```python
from build123d import *

# Parameters (mm, degrees)
SKETCH2_R           = 3
BOSS_EXTRUDE1_DEPTH = 16
CHAMFER1_SIZE       = 1.9304
CHAMFER1_SIZE2      = 10.947842425
FILLET2_R           = 0.7112
SKETCH3_R           = 3.25
BOSS_EXTRUDE2_DEPTH = 2.5
SKETCH4_W           = 71.5000084
SKETCH4_H           = 6.5
BOSS_EXTRUDE3_DEPTH = 0.75
LPATTERN1_START     = 15.124999972
LPATTERN1_OUTLINE_R = 3.25
LPATTERN1_DEPTH     = 0.875000028
SKETCH5_W           = 83
SKETCH5_H           = 9
BOSS_EXTRUDE4_DEPTH = 0.7


# Read off the part's stored shape, not the designer's step: LPattern1
with BuildPart() as part:
    # Sketch2 → Boss-Extrude1 (new body)
    with BuildSketch(Plane(origin=(0, 0, 0), x_dir=(1, 0, 0), z_dir=(0, 1, 0))):
        with Locations(Location((0, 0, 0), (0, 0, 270))):
            Circle(SKETCH2_R)
    extrude(amount=BOSS_EXTRUDE1_DEPTH)

    # Chamfer1
    chamfer1_edges = [part.edges().sort_by_distance(p)[0] for p in [
        (0, 0, -3),
    ]]
    chamfer1_side = [part.faces().sort_by_distance(p)[0] for p in [
        (0, 0, 0),
    ]]
    chamfer(chamfer1_edges, length=CHAMFER1_SIZE, length2=CHAMFER1_SIZE2, reference=chamfer1_side[0])

    # Fillet2
    fillet2_edges = [part.edges().sort_by_distance(p)[0] for p in [
        (0, 0, -1.0696),
    ]]
    fillet(fillet2_edges, radius=FILLET2_R)

    # Sketch3 → Boss-Extrude2 (add)
    with BuildSketch(Plane(origin=(0, 16, 0), x_dir=(1, 0, 0), z_dir=(0, 1, 0))):
        with Locations(Location((0, 0, 0), (0, 0, 270))):
            Circle(SKETCH3_R)
    extrude(amount=-BOSS_EXTRUDE2_DEPTH)

    # Sketch4 → Boss-Extrude3 (add)
    with BuildSketch(Plane(origin=(0, 15.124999972, 0), x_dir=(1, 0, 0), z_dir=(0, 1, 0))):
        with Locations((-31.5000042, 0)):
            Rectangle(SKETCH4_W, SKETCH4_H)
    extrude(amount=-BOSS_EXTRUDE3_DEPTH)

    # LPattern1 outline → LPattern1 (add)
    with BuildSketch(Plane(origin=(0, 0, 0), x_dir=(1, 0, 0), z_dir=(0, 1, 0)).offset(LPATTERN1_START)):
        with Locations((-9, 0)):
            Circle(LPATTERN1_OUTLINE_R)
        with Locations((-18, 0)):
            Circle(LPATTERN1_OUTLINE_R)
        with Locations((-27, 0)):
            Circle(LPATTERN1_OUTLINE_R)
        with Locations((-36, 0)):
            Circle(LPATTERN1_OUTLINE_R)
        with Locations((-45, 0)):
            Circle(LPATTERN1_OUTLINE_R)
        with Locations((-54, 0)):
            Circle(LPATTERN1_OUTLINE_R)
        with Locations((-63, 0)):
            Circle(LPATTERN1_OUTLINE_R)
    extrude(amount=LPATTERN1_DEPTH)

    # LPattern1 2 outline → LPattern1 2 (revolve)
    with BuildSketch(Plane(origin=(-9, 0, 0), x_dir=(1, 0, 0), z_dir=(0, 0, 1))):
        with BuildLine():
            Line((0, 14.374999972), (0, 0))
            Line((0, 0), (0.472832342, 0))
            ThreePointArc((0.472832342, 0), (0.92998289, 0.166389192), (1.173227616, 0.587701416))
            Line((1.173227616, 0.587701416), (3, 10.947842425))
            Line((3, 10.947842425), (3, 13.5))
            Line((3, 13.5), (3.25, 13.5))
            Line((3.25, 13.5), (3.25, 14.374999972))
            Line((3.25, 14.374999972), (0, 14.374999972))
        make_face()
    revolve(axis=Axis((-9, 0, 0), (0, 1, 0)))

    # LPattern1 3 outline → LPattern1 3 (revolve)
    with BuildSketch(Plane(origin=(-18, 0, 0), x_dir=(1, 0, 0), z_dir=(0, 0, 1))):
        with BuildLine():
            Line((0, 14.374999972), (0, 0))
            Line((0, 0), (0.472832342, 0))
            ThreePointArc((0.472832342, 0), (0.92998289, 0.166389192), (1.173227616, 0.587701416))
            Line((1.173227616, 0.587701416), (3, 10.947842425))
            Line((3, 10.947842425), (3, 13.5))
            Line((3, 13.5), (3.25, 13.5))
            Line((3.25, 13.5), (3.25, 14.374999972))
            Line((3.25, 14.374999972), (0, 14.374999972))
        make_face()
    revolve(axis=Axis((-18, 0, 0), (0, 1, 0)))

    # LPattern1 4 outline → LPattern1 4 (revolve)
    with BuildSketch(Plane(origin=(-27, 0, 0), x_dir=(1, 0, 0), z_dir=(0, 0, 1))):
        with BuildLine():
            Line((0, 14.374999972), (0, 0))
            Line((0, 0), (0.472832342, 0))
            ThreePointArc((0.472832342, 0), (0.92998289, 0.166389192), (1.173227616, 0.587701416))
            Line((1.173227616, 0.587701416), (3, 10.947842425))
            Line((3, 10.947842425), (3, 13.5))
            Line((3, 13.5), (3.25, 13.5))
            Line((3.25, 13.5), (3.25, 14.374999972))
            Line((3.25, 14.374999972), (0, 14.374999972))
        make_face()
    revolve(axis=Axis((-27, 0, 0), (0, 1, 0)))

    # LPattern1 5 outline → LPattern1 5 (revolve)
    with BuildSketch(Plane(origin=(-36, 0, 0), x_dir=(1, 0, 0), z_dir=(0, 0, 1))):
        with BuildLine():
            Line((0, 14.374999972), (0, 0))
            Line((0, 0), (0.472832342, 0))
            ThreePointArc((0.472832342, 0), (0.92998289, 0.166389192), (1.173227616, 0.587701416))
            Line((1.173227616, 0.587701416), (3, 10.947842425))
            Line((3, 10.947842425), (3, 13.5))
            Line((3, 13.5), (3.25, 13.5))
            Line((3.25, 13.5), (3.25, 14.374999972))
            Line((3.25, 14.374999972), (0, 14.374999972))
        make_face()
    revolve(axis=Axis((-36, 0, 0), (0, 1, 0)))

    # LPattern1 6 outline → LPattern1 6 (revolve)
    with BuildSketch(Plane(origin=(-45, 0, 0), x_dir=(1, 0, 0), z_dir=(0, 0, 1))):
        with BuildLine():
            Line((0, 14.374999972), (0, 0))
            Line((0, 0), (0.472832342, 0))
            ThreePointArc((0.472832342, 0), (0.92998289, 0.166389192), (1.173227616, 0.587701416))
            Line((1.173227616, 0.587701416), (3, 10.947842425))
            Line((3, 10.947842425), (3, 13.5))
            Line((3, 13.5), (3.25, 13.5))
            Line((3.25, 13.5), (3.25, 14.374999972))
            Line((3.25, 14.374999972), (0, 14.374999972))
        make_face()
    revolve(axis=Axis((-45, 0, 0), (0, 1, 0)))

    # LPattern1 7 outline → LPattern1 7 (revolve)
    with BuildSketch(Plane(origin=(-54, 0, 0), x_dir=(1, 0, 0), z_dir=(0, 0, 1))):
        with BuildLine():
            Line((0, 14.374999972), (0, 0))
            Line((0, 0), (0.472832342, 0))
            ThreePointArc((0.472832342, 0), (0.92998289, 0.166389192), (1.173227616, 0.587701416))
            Line((1.173227616, 0.587701416), (3, 10.947842425))
            Line((3, 10.947842425), (3, 13.5))
            Line((3, 13.5), (3.25, 13.5))
            Line((3.25, 13.5), (3.25, 14.374999972))
            Line((3.25, 14.374999972), (0, 14.374999972))
        make_face()
    revolve(axis=Axis((-54, 0, 0), (0, 1, 0)))

    # LPattern1 8 outline → LPattern1 8 (revolve)
    with BuildSketch(Plane(origin=(-63, 0, 0), x_dir=(1, 0, 0), z_dir=(0, 0, 1))):
        with BuildLine():
            Line((0, 14.374999972), (0, 0))
            Line((0, 0), (0.472832342, 0))
            ThreePointArc((0.472832342, 0), (0.92998289, 0.166389192), (1.173227616, 0.587701416))
            Line((1.173227616, 0.587701416), (3, 10.947842425))
            Line((3, 10.947842425), (3, 13.5))
            Line((3, 13.5), (3.25, 13.5))
            Line((3.25, 13.5), (3.25, 14.374999972))
            Line((3.25, 14.374999972), (0, 14.374999972))
        make_face()
    revolve(axis=Axis((-63, 0, 0), (0, 1, 0)))

    # Sketch5 → Boss-Extrude4 (add)
    with BuildSketch(Plane(origin=(0, 16, 0), x_dir=(1, 0, 0), z_dir=(0, 1, 0))):
        with Locations((-31.5, 0)):
            Rectangle(SKETCH5_W, SKETCH5_H)
    extrude(amount=BOSS_EXTRUDE4_DEPTH)


solid = part.part
```
Geometry check sheet. Reference: the model listing, model coordinates, mm. A direction names the side the tool comes from. Coordinates: 2 decimals unless noted, no trailing zeros. Loops run counter-clockwise (first coordinate to the right, second up) from the corner with the lowest first, then second, coordinate; pieces in that order, holes last. Notation, with made-up numbers: (19.25, 67.25) -> (40.25, 67.25) arc R17 cw to (40.25, 83.25) -> close; hole circle Ø9 at (-12.5, -32). An arc over 180 degrees is marked (long way). Put each result on its own line as item: value.
1) Gauge pin test, flat ends, axial feed: pin 1 Ø8 at (x, y) = (-47, 5.5) entering from -Z; pin 2 Ø5 at (x, z) = (-48.5, 0.5) entering from -Y; pin 3 Ø3 at (x, z) = (0, -1) entering from -Y; pin 4 Ø5 at (y, z) = (6, -1.5) entering from +X. Record the tip position at first contact, or that the pin passes through.
Result set:
pin 1: stops at z = -2.66
pin 2: stops at y = 0.28
pin 3: stops at y = 0
pin 4: stops at x = 2.5
2) Cross-section at A-A on y = 4.5. Record the boundary of the cut face in (x, z).
Result set:
outline: circle Ø3.73 at (-63, 0); circle Ø3.73 at (-54, 0); circle Ø3.73 at (-45, 0); circle Ø3.73 at (-36, 0); circle Ø3.73 at (-27, 0); circle Ø3.73 at (-18, 0); circle Ø3.73 at (-9, 0); circle Ø3.73 at (0, 0)
3) Cross-section at B-B on y = 9. Record the boundary of the cut face in (x, z), plus the area to 3 significant figures.
Result set:
outline: circle Ø5.31 at (-63, 0); circle Ø5.31 at (-54, 0); circle Ø5.31 at (-45, 0); circle Ø5.31 at (-36, 0); circle Ø5.31 at (-27, 0); circle Ø5.31 at (-18, 0); circle Ø5.31 at (-9, 0); circle Ø5.31 at (0, 0)
area: 177 mm^2
4) Release check for a two-part mould opening along X. For faces 1 (the conical face through (-0.8, 5.84, 1.94)), 2 (the flat face through (-67, 14.375, 0)), 3 (the cylindrical face through (0.9, 12.21, 2.86)) record: released by +X, released by -X, zero draft, split by the parting line, or undercut.
Result set:
face 1: undercut
face 2: zero draft
face 3: undercut
5) Thickness scan on line 1 (Y direction, x = -29.5, z = 2.75) (3 decimals); line 2 (Y direction, x = -65, z = -3.5); line 3 (Y direction, x = -48, z = -1). Record the ranges inside material, lowest first.
Result set:
line 1: y = 14.375 to 15.125, 16 to 16.7
line 2: y = 16 to 16.7
line 3: y = 13.5 to 16.7
6) Tool access check on faces 4 (the cylindrical face through (-21.247, 15.556, -0.143)), 5 (the cylindrical face through (-30, 12, 0)), 6 (the flat face through (-67, 15.125, 0)). Record the directions out of +Z, -Z, +X, -X, +Y, -Y that give a thin tool (end or side, any length) a straight path to the whole face; none if there is none.
Result set:
face 4: none
face 5: -Y
face 6: -X
